from build123d import *

# Parameters (mm, degrees)
SKETCH1_R           = 4
BOSS_EXTRUDE1_DEPTH = 52.14
SKETCH2_R           = 6
BOSS_EXTRUDE2_DEPTH = 3
SKETCH3_R           = 0.2
CUT_EXTRUDE1_DEPTH  = 3
CIRPATTERN1_START   = 52.14
CIRPATTERN1_DEPTH   = 3


# Read off the part's stored shape, not the designer's step: CirPattern1
with BuildPart() as part:
    # Sketch1 → Boss-Extrude1 (new body)
    with BuildSketch(Plane(origin=(0, 0, 0), x_dir=(0, 0, -1), z_dir=(1, 0, 0))):
        Circle(SKETCH1_R)
    extrude(amount=BOSS_EXTRUDE1_DEPTH)

    # Sketch2 → Boss-Extrude2 (add)
    with BuildSketch(Plane(origin=(52.14, 0, 0), x_dir=(0, 0, -1), z_dir=(1, 0, 0))):
        Circle(SKETCH2_R)
    extrude(amount=BOSS_EXTRUDE2_DEPTH)

    # Sketch3 → Cut-Extrude1 (cut)
    with BuildSketch(Plane(origin=(55.14, 0, 0), x_dir=(0, 0, -1), z_dir=(1, 0, 0))):
        with Locations((-6, 0)):
            Circle(SKETCH3_R)
    extrude(amount=-CUT_EXTRUDE1_DEPTH, mode=Mode.SUBTRACT)

    # CirPattern1 outline → CirPattern1 (cut)
    with BuildSketch(Plane.YZ.offset(CIRPATTERN1_START)):
        with BuildLine():
            ThreePointArc((-1.358893208, 5.844091824), (-1.552914271, 5.795554958), (-1.745209873, 5.740578586))
            ThreePointArc((-1.745209873, 5.740578586), (-1.501150462, 5.602369792), (-1.358893208, 5.844091824))
        make_face()
        with BuildLine():
            ThreePointArc((1.358893208, 5.844091824), (1.501150462, 5.602369792), (1.745209873, 5.740578586))
            ThreePointArc((1.745209873, 5.740578586), (1.552914271, 5.795554958), (1.358893208, 5.844091824))
        make_face()
        with BuildLine():
            ThreePointArc((2.825152311, 5.293251782), (2.9, 5.022947342), (3.171514356, 5.093279561))
            ThreePointArc((3.171514356, 5.093279561), (3, 5.196152423), (2.825152311, 5.293251782))
        make_face()
        with BuildLine():
            ThreePointArc((4.098881951, 4.381685378), (4.101219331, 4.101219331), (4.381685378, 4.098881951))
            ThreePointArc((4.381685378, 4.098881951), (4.242640687, 4.242640687), (4.098881951, 4.381685378))
        make_face()
        with BuildLine():
            ThreePointArc((5.093279561, 3.171514356), (5.022947342, 2.9), (5.293251782, 2.825152311))
            ThreePointArc((5.293251782, 2.825152311), (5.196152423, 3), (5.093279561, 3.171514356))
        make_face()
        with BuildLine():
            ThreePointArc((5.740578586, 1.745209873), (5.602369792, 1.501150462), (5.844091824, 1.358893208))
            ThreePointArc((5.844091824, 1.358893208), (5.795554958, 1.552914271), (5.740578586, 1.745209873))
        make_face()
        with BuildLine():
            ThreePointArc((5.996666667, 0.19997222), (5.8, 0), (5.996666667, -0.19997222))
            ThreePointArc((5.996666667, -0.19997222), (6, 0), (5.996666667, 0.19997222))
        make_face()
        with BuildLine():
            ThreePointArc((5.844091824, -1.358893208), (5.602369792, -1.501150462), (5.740578586, -1.745209873))
            ThreePointArc((5.740578586, -1.745209873), (5.795554958, -1.552914271), (5.844091824, -1.358893208))
        make_face()
        with BuildLine():
            ThreePointArc((5.293251782, -2.825152311), (5.022947342, -2.9), (5.093279561, -3.171514356))
            ThreePointArc((5.093279561, -3.171514356), (5.196152423, -3), (5.293251782, -2.825152311))
        make_face()
        with BuildLine():
            ThreePointArc((4.381685378, -4.098881951), (4.101219331, -4.101219331), (4.098881951, -4.381685378))
            ThreePointArc((4.098881951, -4.381685378), (4.242640687, -4.242640687), (4.381685378, -4.098881951))
        make_face()
        with BuildLine():
            ThreePointArc((3.171514356, -5.093279561), (2.9, -5.022947342), (2.825152311, -5.293251782))
            ThreePointArc((2.825152311, -5.293251782), (3, -5.196152423), (3.171514356, -5.093279561))
        make_face()
        with BuildLine():
            ThreePointArc((1.745209873, -5.740578586), (1.501150462, -5.602369792), (1.358893208, -5.844091824))
            ThreePointArc((1.358893208, -5.844091824), (1.552914271, -5.795554958), (1.745209873, -5.740578586))
        make_face()
        with BuildLine():
            ThreePointArc((0.19997222, -5.996666667), (0, -5.8), (-0.19997222, -5.996666667))
            ThreePointArc((-0.19997222, -5.996666667), (0, -6), (0.19997222, -5.996666667))
        make_face()
        with BuildLine():
            ThreePointArc((-1.358893208, -5.844091824), (-1.501150462, -5.602369792), (-1.745209873, -5.740578586))
            ThreePointArc((-1.745209873, -5.740578586), (-1.552914271, -5.795554958), (-1.358893208, -5.844091824))
        make_face()
        with BuildLine():
            ThreePointArc((-2.825152311, -5.293251782), (-2.9, -5.022947342), (-3.171514356, -5.093279561))
            ThreePointArc((-3.171514356, -5.093279561), (-3, -5.196152423), (-2.825152311, -5.293251782))
        make_face()
        with BuildLine():
            ThreePointArc((-4.098881951, -4.381685378), (-4.101219331, -4.101219331), (-4.381685378, -4.098881951))
            ThreePointArc((-4.381685378, -4.098881951), (-4.242640687, -4.242640687), (-4.098881951, -4.381685378))
        make_face()
        with BuildLine():
            ThreePointArc((-5.093279561, -3.171514356), (-5.022947342, -2.9), (-5.293251782, -2.825152311))
            ThreePointArc((-5.293251782, -2.825152311), (-5.196152423, -3), (-5.093279561, -3.171514356))
        make_face()
        with BuildLine():
            ThreePointArc((-5.740578586, -1.745209873), (-5.602369792, -1.501150462), (-5.844091824, -1.358893208))
            ThreePointArc((-5.844091824, -1.358893208), (-5.795554958, -1.552914271), (-5.740578586, -1.745209873))
        make_face()
        with BuildLine():
            ThreePointArc((-5.996666667, -0.19997222), (-5.8, 0), (-5.996666667, 0.19997222))
            ThreePointArc((-5.996666667, 0.19997222), (-6, 0), (-5.996666667, -0.19997222))
        make_face()
        with BuildLine():
            ThreePointArc((-5.844091824, 1.358893208), (-5.602369792, 1.501150462), (-5.740578586, 1.745209873))
            ThreePointArc((-5.740578586, 1.745209873), (-5.795554958, 1.552914271), (-5.844091824, 1.358893208))
        make_face()
        with BuildLine():
            ThreePointArc((-5.293251782, 2.825152311), (-5.022947342, 2.9), (-5.093279561, 3.171514356))
            ThreePointArc((-5.093279561, 3.171514356), (-5.196152423, 3), (-5.293251782, 2.825152311))
        make_face()
        with BuildLine():
            ThreePointArc((-4.381685378, 4.098881951), (-4.101219331, 4.101219331), (-4.098881951, 4.381685378))
            ThreePointArc((-4.098881951, 4.381685378), (-4.242640687, 4.242640687), (-4.381685378, 4.098881951))
        make_face()
        with BuildLine():
            ThreePointArc((-3.171514356, 5.093279561), (-2.9, 5.022947342), (-2.825152311, 5.293251782))
            ThreePointArc((-2.825152311, 5.293251782), (-3, 5.196152423), (-3.171514356, 5.093279561))
        make_face()
    extrude(amount=CIRPATTERN1_DEPTH, mode=Mode.SUBTRACT)


solid = part.part
Could you check a few things on this model? Use its own coordinates, in mm. Give positions to 0.01 mm unless a question says otherwise; leave off trailing zeros. Order: outer loops, then holes, each group sorted by start corner. A loop starts at its lowest first (then second) coordinate and runs counter-clockwise, first axis right, second up. Notation, with made-up numbers: (-39, 6) - (18, 6) arc R4 cw to (18, 10) - close; hole circle Ø11 at (23, -5.5). An arc over 180 degrees is marked (long way). One line per question, with ' | ' between items. Start each with the question number.
Item 1: I want a section at A-A on y = -2.25. Write out the boundary of the cut face in (x, z), then the cut area to 3 significant figures.
Item 2: I'm going to push flat-ended pins straight in: pin 1 Ø6 at (x, y) = (19, 3.5) entering from +Z; pin 2 Ø1.5 at (x, z) = (34.5, 2.5) entering from +Y; pin 3 Ø4 at (x, y) = (40.5, 3.5) entering from -Z. Where does each tip first touch, or does it pass through?
Item 3: I need wall thicknesses on probe 1 along X at (y, z) = (-4.75, -2); probe 2 along Z at (x, y) = (10.5, 1.5); probe 3 along Z at (x, y) = (25, -0.25). Which ranges of each line are inside material? Lowest first, please. Write a range as [from, to].
Item 4: I want a section at B-B on x = 30.5. Write out the boundary of the cut face in (y, z).
Item 5: Thinking about a two-plate mould opening in X: for faces 1 (the cylindrical face through (53.619, -5.948, 0.791)), 2 (the flat face through (55.14, 0, 0)), which applies, pulls with the +X half, pulls with the -X half, needs draft (parallel to the pull), parting line crosses it, or undercut?
Verdict:
1) outline: (0, -3.31) - (52.14, -3.31) - (52.14, -5.56) - (55.14, -5.56) - (55.14, 5.56) - (52.14, 5.56) - (52.14, 3.31) - (0, 3.31) - close | area: 378 mm^2
2) pin 1: z = 3.97 | pin 2: y = 3.6 | pin 3: z = -3.71
3) probe 1: [52.14, 55.14] | probe 2: [-3.71, 3.71] | probe 3: [-3.99, 3.99]
4) outline: circle Ø8 at (0, 0)
5) face 1: needs draft | face 2: pulls with the +X half
